from build123d import *

# Parameters (mm, degrees)
SKETCH1_W           = 254
SKETCH1_H           = 50.8
BOSS_EXTRUDE1_DEPTH = 4.699
SKETCH2_W           = 203.2
SKETCH2_H           = 7.62
CUT_EXTRUDE1_DEPTH  = 381.549968508
CAVITY1_START       = 125.842884167
CAVITY1_OUTLINE_W   = 4.699
CAVITY1_OUTLINE_H   = 4.699
CAVITY1_DEPTH       = 44.45
CAVITY1_START_2     = 214.742884167
CAVITY1_2_OUTLINE_W = 4.699
CAVITY1_2_OUTLINE_H = 4.699
CAVITY1_2_DEPTH     = 44.45
CAVITY1_START_3     = 303.642884167
CAVITY1_3_OUTLINE_W = 4.699
CAVITY1_3_OUTLINE_H = 4.699
CAVITY1_3_DEPTH     = 31.75


# Read off the part's stored shape, not the designer's step: Cavity1
with BuildPart() as part:
    # Sketch1 → Boss-Extrude1 (new body)
    with BuildSketch(Plane.XY):
        with Locations((208.392884167, -154.343737527)):
            Rectangle(SKETCH1_W, SKETCH1_H)
    extrude(amount=BOSS_EXTRUDE1_DEPTH)

    # Sketch2 → Cut-Extrude1 (cut, through all)
    with BuildSketch(Plane(origin=(0, 0, 0), x_dir=(-1, 0, 0), z_dir=(0, 0, -1))):
        with Locations((-208.392884167, -154.343737527)):
            Rectangle(SKETCH2_W, SKETCH2_H)
    extrude(amount=-CUT_EXTRUDE1_DEPTH, mode=Mode.SUBTRACT)

    # Cavity1 outline → Cavity1 (cut)
    with BuildSketch(Plane.YZ.offset(CAVITY1_START)):
        with Locations((-177.394237527, 2.3495)):
            Rectangle(CAVITY1_OUTLINE_W, CAVITY1_OUTLINE_H)
        with Locations((-131.293237527, 2.3495)):
            Rectangle(CAVITY1_OUTLINE_W, CAVITY1_OUTLINE_H)
    extrude(amount=CAVITY1_DEPTH, mode=Mode.SUBTRACT)

    # Cavity1 2 outline → Cavity1 2 (cut)
    with BuildSketch(Plane.YZ.offset(CAVITY1_START_2)):
        with Locations((-177.394237527, 2.3495)):
            Rectangle(CAVITY1_2_OUTLINE_W, CAVITY1_2_OUTLINE_H)
        with Locations((-131.293237527, 2.3495)):
            Rectangle(CAVITY1_2_OUTLINE_W, CAVITY1_2_OUTLINE_H)
    extrude(amount=CAVITY1_2_DEPTH, mode=Mode.SUBTRACT)

    # Cavity1 3 outline → Cavity1 3 (cut)
    with BuildSketch(Plane.YZ.offset(CAVITY1_START_3)):
        with Locations((-177.394237527, 2.3495)):
            Rectangle(CAVITY1_3_OUTLINE_W, CAVITY1_3_OUTLINE_H)
        with Locations((-131.293237527, 2.3495)):
            Rectangle(CAVITY1_3_OUTLINE_W, CAVITY1_3_OUTLINE_H)
    extrude(amount=CAVITY1_3_DEPTH, mode=Mode.SUBTRACT)


solid = part.part
CAD build for the part. Positions are in the model's coordinates, mm. A direction names the side the tool comes from. Give positions to 0.01 mm unless a question says otherwise; leave off trailing zeros. Order: outer loops, then holes, each group sorted by start corner. A loop starts at its lowest first (then second) coordinate and runs counter-clockwise, first axis right, second up. Notation, with made-up numbers: (76, 12.5) -> (128, 12.5) arc R26 ccw to (128, 50.5) -> close; hole circle Ø6 at (34, 29.25). An arc over 180 degrees is marked (long way). Return JSON: item names as keys, results as strings.
Q1. Flat gauge pins, fed straight in: pin 1 (5 mm diameter, centred on x = 211, y = -156, fed in from -Z); pin 2 (1.4 mm diameter, centred on x = 139, z = 2, fed in from -Y); pin 3 (1.4 mm diameter, centred on y = -130.5, z = 1, fed in from +X); pin 4 (1.4 mm diameter, centred on x = 157.5, z = 2.5, fed in from +Y). Where does each tip first touch, or does it go through?
Working result:
{"pin 1": "z = 0", "pin 2": "y = -175.04", "pin 3": "x = 303.64", "pin 4": "y = -133.64"}
Q2. Mould opens along X. For faces 4 (the face through (207, -160, 4.699)), 5 (the face through (237, -175.045, 2)), 6 (the face through (335.393, -155, 2)) say: pulls with the +X half, pulls with the -X half, needs draft (parallel to the pull), parting line crosses it, or undercut.
Working result:
{"face 4": "needs draft", "face 5": "undercut", "face 6": "pulls with the +X half"}
Q3. Drill centre lines: line 1 (X direction, y = -130.5, z = 1.6); line 2 (X direction, y = -151, z = 1.3); line 3 (Y direction, x = 244, z = 4.2). Where is each one in solid material? Low to high.
Working result:
{"line 1": "81.39 to 125.84, 170.29 to 214.74, 259.19 to 303.64", "line 2": "81.39 to 106.79, 309.99 to 335.39", "line 3": "-175.04 to -158.15, -150.53 to -133.64"}
Q4. Saw through at A-A (z = 2.55). Write the cut outline in (x, y).
Working result:
{"outline": "(81.39, -179.74) -> (125.84, -179.74) -> (125.84, -175.04) -> (170.29, -175.04) -> (170.29, -179.74) -> (214.74, -179.74) -> (214.74, -175.04) -> (259.19, -175.04) -> (259.19, -179.74) -> (303.64, -179.74) -> (303.64, -175.04) -> (335.39, -175.04) -> (335.39, -133.64) -> (303.64, -133.64) -> (303.64, -128.94) -> (259.19, -128.94) -> (259.19, -133.64) -> (214.74, -133.64) -> (214.74, -128.94) -> (170.29, -128.94) -> (170.29, -133.64) -> (125.84, -133.64) -> (125.84, -128.94) -> (81.39, -128.94) -> close; hole (106.79, -158.15) -> (309.99, -158.15) -> (309.99, -150.53) -> (106.79, -150.53) -> close"}
Q5. Saw through at C-C (x = 221.5). Write the cut outline in (y, z).
Working result:
{"outline": "(-175.04, 0) -> (-158.15, 0) -> (-158.15, 4.7) -> (-175.04, 4.7) -> close; (-150.53, 0) -> (-133.64, 0) -> (-133.64, 4.7) -> (-150.53, 4.7) -> close"}
Q6. Saw through at B-B (x = 189.5). Write the cut outline in (y, z).
Working result:
{"outline": "(-179.74, 0) -> (-158.15, 0) -> (-158.15, 4.7) -> (-179.74, 4.7) -> close; (-150.53, 0) -> (-128.94, 0) -> (-128.94, 4.7) -> (-150.53, 4.7) -> close"}
Q7. Which spindle directions (+Z, -Z, +X, -X, +Y, -Y) get a long thin tool onto all of the face, cutting with end or side? Do faces 1 (the face through (125.843, -177, 2)), 2 (the face through (237, -133.643, 2)), 3 (the face through (210, -150.534, 2)). Say none if no direction does.
Working result:
{"face 1": "+Z, -Z, -Y", "face 2": "+Z, -Z, +Y", "face 3": "+Z, -Z"}
